```python
from build123d import *

# Parameters (mm, degrees)
F0_R            = 62.5
F1_DEPTH        = 10
F2_R            = 3
F3_DEPTH        = 125
F3_COPIES_COUNT = 8
F4_R            = 8
F5_DEPTH        = 120


# Not quite as in the source:
# - a pattern or mirror of a feature is missing from the dataset's text; its kind, count and spacing are read off the source's solid


with BuildPart() as f1:
    # F0 (on Top) → F1 (new body)
    with BuildSketch(Plane.XY):
        Circle(F0_R)
    extrude(amount=F1_DEPTH)

    # F2 (on face) → F3 (join)
    with BuildSketch(Plane.XY.offset(10)):
        with Locations((10, 0)):
            Circle(F2_R)
        with Locations((20, 0)):
            Circle(F2_R)
        with Locations((30, 0)):
            Circle(F2_R)
        with Locations((40, 0)):
            Circle(F2_R)
        with Locations((50, 0)):
            Circle(F2_R)
    f3 = extrude(amount=F3_DEPTH)

    # F3_copies: F3 ×8 about axis
    f3_copies_axis = Axis((0, 0, 0), (0, 0, 1))
    for i in range(1, F3_COPIES_COUNT):
        add(f3.rotate(f3_copies_axis, i * 360 / F3_COPIES_COUNT))

    # F4 (on face) → F5 (join)
    with BuildSketch(Plane.XY):
        Circle(F4_R)
    extrude(amount=-F5_DEPTH)


solid = f1.part
```
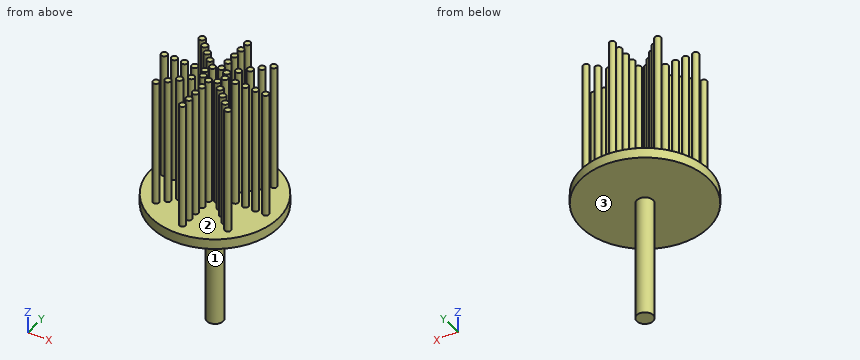
Build history of the part. All positions in model axes, mm. Face numbers are marked on the shaded views. Coordinates: 2 decimals unless noted, no trailing zeros. Order: outer loops, then holes, each group sorted by start corner. A loop starts at its lowest first (then second) coordinate and runs counter-clockwise, first axis right, second up.
Item 1: Saw through at A-A on y = 50. List the corners of the cut face in (x, z), then the cut area to 3 significant figures.
Filled in:
outline: (-37.5, 0) - (37.5, 0) - (37.5, 10) - (3, 10) - (3, 135) - (-3, 135) - (-3, 10) - (-37.5, 10) - close
area: 1,500 mm2
Item 2: Drill centre lines: L1, parallel to X at y = -28, z = 104; L2, parallel to Y at x = 12, z = 99; L3, parallel to Z at x = 8, y = -48. Where is each one in solid material? Low to high.
Filled in:
L1: x = -31.27 to -25.3, -2.24 to 2.24, 25.3 to 31.27
L2: y = -16.24 to -12.04, -2.24 to 2.24, 12.04 to 16.24
L3: z = 0 to 10
Item 3: Saw through at C-C on z = -95. List the corners of the cut face in (x, y), then the cut area to 3 significant figures.
Filled in:
outline: circle Ø16 at (0, 0)
area: 201 mm2
Item 4: Mould opens along Y. For the marked faces 1, 2 and 3 say: released by +Y, released by -Y, zero draft, split by the parting line, or undercut.
Filled in:
face 1: split by the parting line
face 2: undercut
face 3: zero draft
Item 5: Drop flat-ended pins along their axis: pin 1 Ø1.5 at (x, y) = (-41, 28.5) entering from -Z; pin 2 Ø10 at (x, z) = (-47, 79) entering from -Y; pin 3 Ø12 at (x, y) = (-14.5, 7) entering from +Z; pin 4 Ø1.5 at (x, z) = (9.5, 74) entering from -Y. Give the stop position or say it passes through.
Filled in:
pin 1: stops at z = 0
pin 2: stops at y = -3
pin 3: stops at z = 135
pin 4: stops at y = -9.56
